from build123d import *

# Parameters (mm, degrees)
F0_W     = 69.122039
F0_H     = 35.963256
F1_DEPTH = 4.826
F2_R     = 5.08
F3_R     = 5.08
F4_R     = 2.639502
F5_DEPTH = 25.4


with BuildPart() as f1:
    # F0 (on Top) → F1 (new body)
    with BuildSketch(Plane.XY):
        with Locations((-34.56102, 17.981628)):
            Rectangle(F0_W, F0_H)
    extrude(amount=F1_DEPTH)

    # F2
    f2_edges = [f1.edges().sort_by_distance(p)[0] for p in [
        (-69.122039, 0, 2.413),
    ]]
    fillet(f2_edges, radius=F2_R)

    # F3
    f3_edges = [f1.edges().sort_by_distance(p)[0] for p in [
        (-69.122039, 35.963256, 2.413),
    ]]
    fillet(f3_edges, radius=F3_R)

    # F4 (on face) → F5 (cut)
    with BuildSketch(Plane.XY.offset(4.826)):
        with Locations((-6.361922, 5.802391)):
            Circle(F4_R)
    extrude(amount=-F5_DEPTH, mode=Mode.SUBTRACT)


solid = f1.part
Source: CAD feature listing. Evaluate the final solid. Frame: model axes, mm. Round coordinates to 2 decimals unless told otherwise and drop trailing zeros. Order: outer loops, then holes, each group sorted by start corner. A loop starts at its lowest first (then second) coordinate and runs counter-clockwise, first axis right, second up. Notation, with made-up numbers: (23, -36) - (66, -36) arc R21 cw to (66, -25) - close; hole circle Ø8 at (69, 81). An arc over 180 degrees is marked (long way). Use a Markdown table: item, result. Add a question column.
1. Section query B-B (y = 7.5). Return the cut outline in (x, z), then the cut area to 3 significant figures.
2. Mould query, pull axis X, two halves, no side actions, for faces 1 (the flat face through (-69.122, 18, 2)), 2 (the flat face through (0, 18, 2)), 3 (the cylindrical face through (-4.9, 8, 2.4)), 4 (the flat face through (-35, 18, 0)). Classes: +X half, -X half, draft (parallel to the pull), parting line (faces both ways), or undercut.
3. Section query A-A (x = -8). Return the cut outline in (y, z).
4. Line query: probe 1 along Y at (x, z) = (-6.5, 4.05); probe 2 along X at (y, z) = (4, 2.8); probe 3 along X at (y, z) = (3.5, 4.4). Output: solid intervals per line, ascending.
Derived:
| question | item | result |
|---|---|---|
| 1 | outline | (-69.12, 0) - (-8.38, 0) - (-8.38, 4.83) - (-69.12, 4.83) - close; (-4.34, 0) - (0, 0) - (0, 4.83) - (-4.34, 4.83) - close |
| 1 | area | 314 mm2 |
| 2 | face 1 | -X half |
| 2 | face 2 | +X half |
| 2 | face 3 | undercut |
| 2 | face 4 | draft |
| 3 | outline | (0, 0) - (3.73, 0) - (3.73, 4.83) - (0, 4.83) - close; (7.87, 0) - (35.96, 0) - (35.96, 4.83) - (7.87, 4.83) - close |
| 4 | probe 1 | 0 to 3.17, 8.44 to 35.96 |
| 4 | probe 2 | -69.01 to -8.29, -4.43 to 0 |
| 4 | probe 3 | -68.87 to -7.65, -5.07 to 0 |
